Part print with two shaded views. Sizes in mm from the minimum x, y, z corner. Give positions to 0.01 mm unless a question says otherwise; leave off trailing zeros. Write each loop counter-clockwise with the first axis right and the second up, starting at its lowest first coordinate (ties: lowest second). Pieces come first, ordered by that corner, then holes. Notation, with made-up numbers: (58.25, 27) -> (113.25, 27) arc R19 cw to (113.25, 51) -> close; hole circle Ø4 at (35, 26.5). An arc over 180 degrees is marked (long way). Answer in a Markdown table with one row per item. Add a question column.
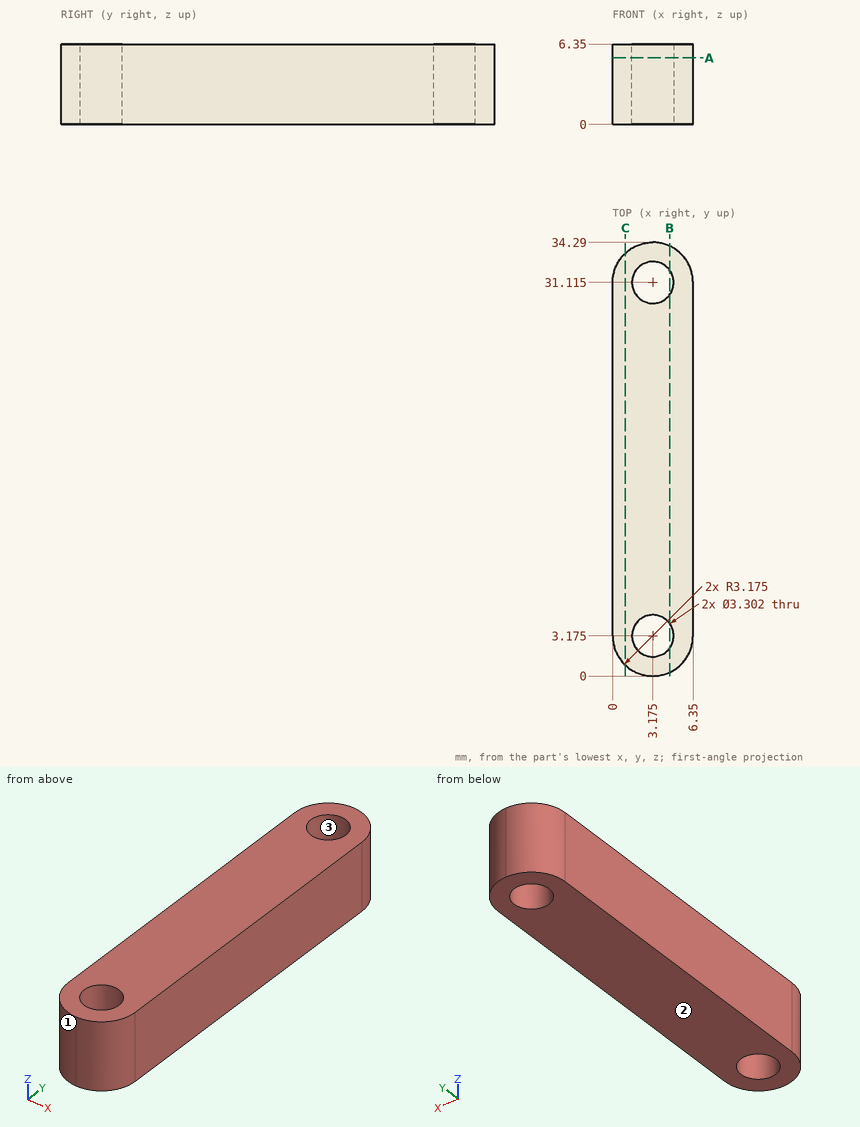
Item 1: Slice it at B-B, the plane x = 4.5. List the corners of the cut face in (y, z).
Item 2: Drop a flat-ended pin along its axis: pin 1 Ø2.5 at (x, y) = (3.175, 31.115) entering from -Z. Give the stop position or say it passes through.
Item 3: Probe L1, parallel to Y at x = 3.25, z = 0.5; L2, parallel to Y at x = 3.75, z = 4.5; L3, parallel to X at y = 3, z = 5.75. List the from-to ranges inside material, lowest first. Write a range as from..to.
Item 4: Slice it at C-C, the plane x = 1. List the corners of the cut face in (y, z).
Item 5: Mould opens along X. For the marked faces 1, 2 and 3 say: released by +X, released by -X, zero draft, split by the parting line, or undercut.
Item 6: Slice it at A-A, the plane z = 5.25. State how many separate pieces and enclosed holes the cut face has, then the cut area to 3 significant figures.
Answer key:
| question | item | result |
|---|---|---|
| 1 | outline | (0.29, 0) -> (2.19, 0) -> (2.19, 6.35) -> (0.29, 6.35) -> close; (4.16, 0) -> (30.13, 0) -> (30.13, 6.35) -> (4.16, 6.35) -> close; (32.1, 0) -> (34, 0) -> (34, 6.35) -> (32.1, 6.35) -> close |
| 2 | pin 1 | passes through |
| 3 | L1 | y = 0..1.53, 4.82..29.47, 32.76..34.29 |
| 3 | L2 | y = 0.05..1.63, 4.72..29.57, 32.66..34.24 |
| 3 | L3 | x = 0..1.53, 4.82..6.35 |
| 4 | outline | (0.86, 0) -> (33.43, 0) -> (33.43, 6.35) -> (0.86, 6.35) -> close |
| 5 | face 1 | released by -X |
| 5 | face 2 | zero draft |
| 5 | face 3 | undercut |
| 6 | separate pieces | 1 |
| 6 | enclosed holes | 2 |
| 6 | area | 192 mm² |
